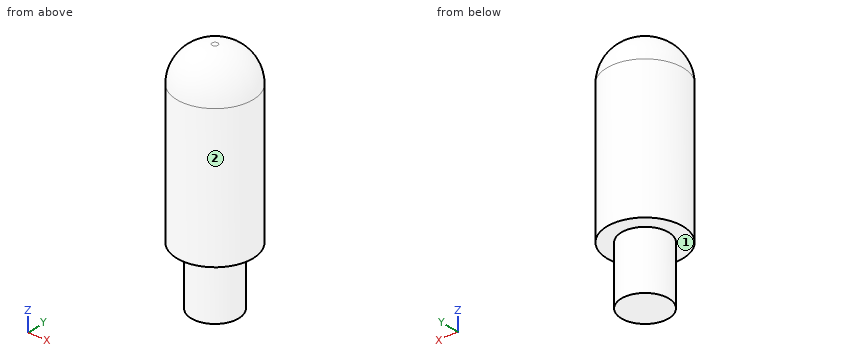
```python
from build123d import *

# Parameters (mm, degrees)
ESQUISSE1_R        = 6.5
BOSS_EXTRU_1_DEPTH = 30
ESQUISSE2_R        = 4.05
BOSS_EXTRU_2_DEPTH = 10
CONG_4_R           = 6


with BuildPart() as part:
    # Esquisse1 → Boss.-Extru.1 (new body)
    with BuildSketch(Plane.XY):
        Circle(ESQUISSE1_R)
    extrude(amount=BOSS_EXTRU_1_DEPTH)

    # Esquisse2 → Boss.-Extru.2 (add)
    with BuildSketch(Plane(origin=(0, 0, 0), x_dir=(-1, 0, 0), z_dir=(0, 0, -1))):
        Circle(ESQUISSE2_R)
    extrude(amount=BOSS_EXTRU_2_DEPTH)

    # Congé4
    cong_4_edges = [part.edges().sort_by_distance(p)[0] for p in [
        (-6.5, 0, 30),
    ]]
    fillet(cong_4_edges, radius=CONG_4_R)


solid = part.part
```
For this review, take the finished solid that the model builds, in its own axes (mm). Face numbers are marked on the shaded views. A direction names the side the tool comes from. Round coordinates to 2 decimals unless told otherwise and drop trailing zeros. Order: outer loops, then holes, each group sorted by start corner. A loop starts at its lowest first (then second) coordinate and runs counter-clockwise, first axis right, second up. Notation, with made-up numbers: (-35.5, 18) -> (-23.5, 18) arc R28 cw to (-23.5, 39) -> close; hole circle Ø7 at (68.5, 2). An arc over 180 degrees is marked (long way). Use a Markdown table: item, result.
Item 1: Take a section at B-B (z = 3). State the section outline as (x, y) points.
Resolved:
| item | result |
|---|---|
| outline | circle Ø13 at (0, 0) |
Item 2: For pin 1 (2 mm diameter, centred on x = -4.5, y = -4.5, fed in from -Z); pin 2 (6 mm diameter, centred on y = 0, z = 25.5, fed in from -X); pin 3 (5 mm diameter, centred on x = 3.5, y = 1, fed in from +Z); pin 4 (1 mm diameter, centred on x = -3, y = 4, fed in from +Z), all flat-tipped, find the tip position at first contact; note any pin that passes through.
Resolved:
| item | result |
|---|---|
| pin 1 | stops at z = 0 |
| pin 2 | stops at x = -6.5 |
| pin 3 | stops at z = 29.97 |
| pin 4 | stops at z = 28.47 |
Item 3: For line 1 along X through (y, z) = (0.25, 12.5); line 2 along X through (y, z) = (1.5, -1.5); line 3 along Y through (x, z) = (2, 13.5), list the stretches that pass through material, from the lowest coordinate up. Write a range as [from, to].
Resolved:
| item | result |
|---|---|
| line 1 | x = [-6.5, 6.5] |
| line 2 | x = [-3.76, 3.76] |
| line 3 | y = [-6.18, 6.18] |
Item 4: Machinability: for the marked faces 1 and 2, which of the approach directions +Z, -Z, +X, -X, +Y, -Y give a long, thin tool a straight path to every point of the face, cutting with its end or side? Answer none if there is none.
Resolved:
| item | result |
|---|---|
| face 1 | -Z |
| face 2 | +Z, -Z |
Item 5: Take a section at A-A (z = -3). State the section outline as (x, y) points, plus the area to 3 significant figures.
Resolved:
| item | result |
|---|---|
| outline | circle Ø8.1 at (0, 0) |
| area | 51.5 mm² |
